Part print with two shaded views. Sizes in mm from the minimum x, y, z corner. A direction names the side the tool comes from. Round coordinates to 2 decimals unless told otherwise and drop trailing zeros. Write each loop counter-clockwise with the first axis right and the second up, starting at its lowest first coordinate (ties: lowest second). Pieces come first, ordered by that corner, then holes. Notation, with made-up numbers: (-5, 0.25) - (12, 0.25) arc R13 cw to (12, 25.25) - close; hole circle Ø7 at (83.25, 53). An arc over 180 degrees is marked (long way). Use one line per item in the form item = value. Start each with the question number.
Item 1: Pin check, flat tips, straight feed: pin 1 (1 mm diameter, centred on y = 8, z = 32, fed in from +X); pin 2 (6 mm diameter, centred on y = 4, z = 13.5, fed in from -X); pin 3 (5 mm diameter, centred on y = 6, z = 42.5, fed in from +X). Stop position of each tip, or through.
Item 2: Pull direction Z, two halves, no side cores. Call the marked faces 3, 4 and 5: +Z half, -Z half, draft (parallel to the pull), parting line (faces both ways), or undercut.
Item 3: Band-saw the part on A-A, the plane x = 25. List the corners of the cut face in (y, z) (1 decimal).
Item 4: Band-saw the part on C-C, the plane y = 2. List the corners of the cut face in (x, z), and give its area (3 significant figures).
Item 5: Drill centre lines: L1, parallel to Z at x = 21, y = 1.5; L2, parallel to Z at x = 25, y = 5.25 (1 decimal); L3, parallel to X at y = 9.75, z = 33 (1 decimal). Where is each one in solid material? Low to high.
Item 6: Tool access for the marked faces 1 and 2: list every direction of +Z, -Z, +X, -X, +Y, -Y with a clear straight run to the whole face (end or side of a thin tool).
Item 7: Band-saw the part on D-D, the plane x = 46. List the corners of the cut face in (y, z) (1 decimal), and give its area (3 significant figures).
Item 8: Band-saw the part on B-B, the plane z = 25. List the corners of the cut face in (x, y).
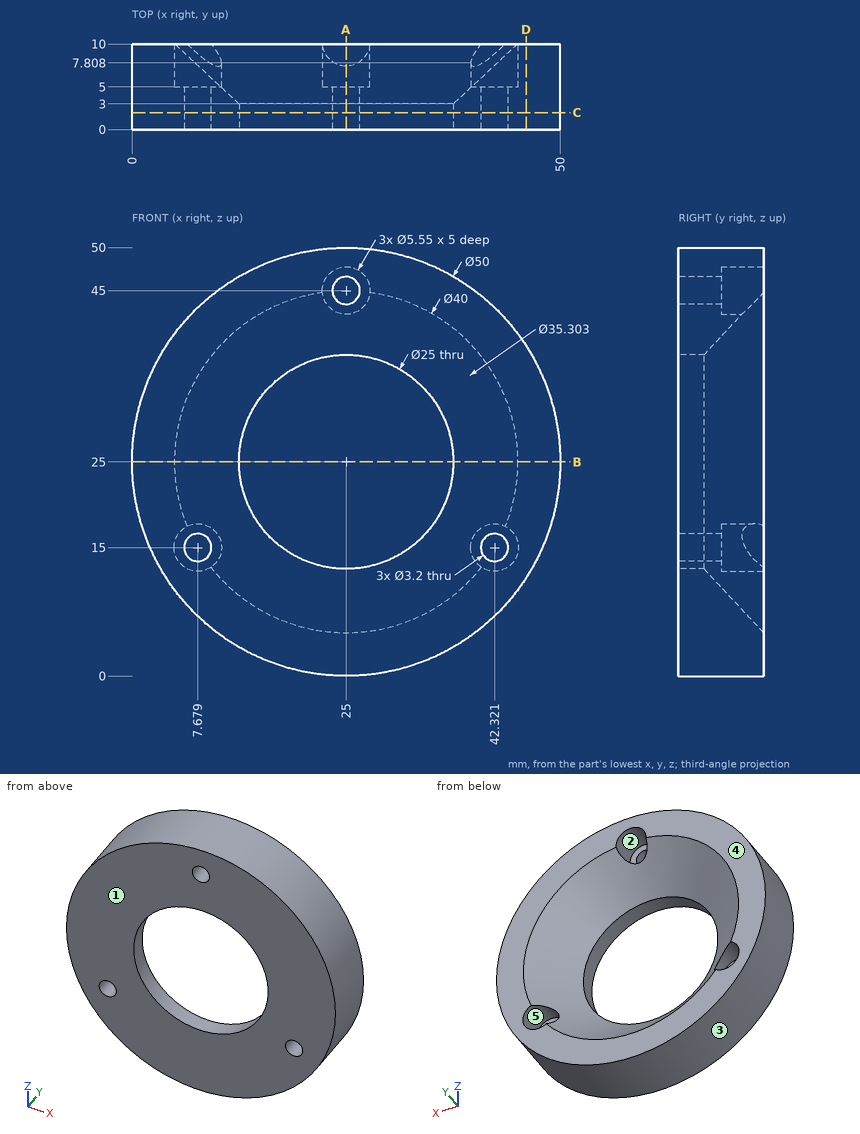
Determined:
q1.pin_1 = 49.14
q1.pin_2 = 1.49
q1.pin_3 = 45
q2.face_3 = parting line
q2.face_4 = draft
q2.face_5 = undercut
q3.outline = (0, 0) - (10, 0) - (10, 5) - (3, 12.5) - (0, 12.5) - close; (0, 37.5) - (3, 37.5) - (7.4, 42.2) - (5, 42.2) - (5, 43.4) - (0, 43.4) - close; (0, 46.6) - (5, 46.6) - (5, 47.8) - (10, 47.8) - (10, 50) - (0, 50) - close
q4.outline = circle Ø50 at (25, 25); hole circle Ø3.2 at (7.68, 15); hole circle Ø25 at (25, 25); hole circle Ø3.2 at (25, 45); hole circle Ø3.2 at (42.32, 15)
q4.area = 1,450 mm²
q5.L1 = 0.32 to 13.16, 36.84 to 49.68
q5.L2 = 0 to 10.1, 39.9 to 42.2, 47.8 to 50
q5.L3 = 1.3 to 7, 43 to 48.7
q6.face_1 = +Z, -Z, +X, -X, -Y
q6.face_2 = +Y
q7.outline = (0, 11.4) - (10, 11.4) - (10, 38.6) - (0, 38.6) - close
q7.area = 271 mm²
q8.outline = (0, 0) - (12.5, 0) - (12.5, 3) - (5, 10) - (0, 10) - close; (37.5, 0) - (50, 0) - (50, 10) - (45, 10) - (37.5, 3) - close
